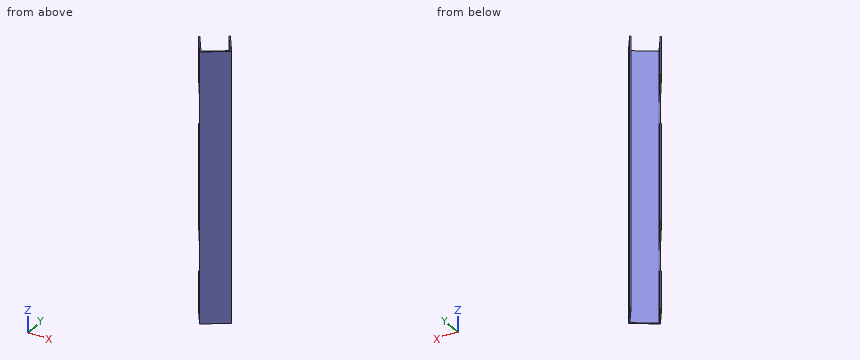
Autodesk Inventor part; units mm, degrees
ref_plane "YZ Plane" through (0, 0, 0) normal (1, 0, 0) x (0, 1, 0)
ref_plane "XZ Plane" through (0, 0, 0) normal (0, 1, 0) x (-1, 0, 0)
ref_plane "XY Plane" through (0, 0, 0) normal (0, 0, 1) x (1, 0, 0)
sketch "Sketch1" plane through (0, 0, 0) normal (0, 0, 1) x (1, 0, 0)
  line L0 (39.1036, 49.5244) -> (75.147, -2.7549)
  line L1 (75.147, -2.7549) -> (22.8678, -38.7983)
  line L2 (22.8678, -38.7983) -> (-13.1757, 13.4809)
  line L3 (41.7176, 51.3265) -> (79.5632, -3.5667)
  line L4 (79.5632, -3.5667) -> (22.056, -43.2145)
  line L5 (22.056, -43.2145) -> (-15.7896, 11.6787)
  line L6 (-13.1757, 13.4809) -> (-15.7896, 11.6787)
  line L7 (41.7176, 51.3265) -> (39.1036, 49.5244)
  point P0 (0, 0)
  dimension "d0" = 63.5
  dimension "d1" = 63.5
  dimension "d2" = 63.5
  dimension "d3" = 3.175
extrude "Extrusion1" add sketch "Sketch1" along normal blind 685.8
sketch "Sketch2" plane through (22.056, -43.2145, 0) normal (-0.8232952, -0.5676134, 0) x (0, 0, 1)
  line L0 (0, 66.675) -> (0, 0)
  line L1 (0, 0) -> (685.8, 0)
  line L2 (685.8, 66.675) -> (685.8, 0)
  line L3 (0, 66.675) -> (685.8, 66.675)
  ellipse E0 centre (510.7417, -1678.7212) end of major axis (489.6597, -1678.7212) minor radius 19.9414
  line L4 (0, 3.175) -> (685.8, 3.175)
  line L5 (568.7405, 20.5903) -> (590.2302, 66.675)
  line L6 (0, 66.675) -> (685.8, 66.675)
  line L7 (466.6953, 66.675) -> (590.2302, 66.675)
  line L8 (508, 66.675) -> (177.8, 66.675) construction
  line L9 (177.8, 20.6195) -> (508, 20.6195) construction
  line L10 (508, 20.6195) -> (558.8, 20.6195) construction
  line L11 (558.8, 20.6195) -> (558.8, 66.675) construction
  line L12 (558.8, 66.675) -> (508, 66.675) construction
  line L13 (508, 66.675) -> (508, 20.6195) construction
  line L14 (466.6953, 66.675) -> (488.7774, 20.3572)
  arc A0 (488.6539, 20.6195) -> (516.004, 3.175) centre (516.004, 33.3375) ccw
  line L15 (541.404, 3.175) -> (516.004, 3.175)
  line L16 (0, 3.175) -> (685.8, 3.175)
  arc A1 (541.404, 3.175) -> (568.7405, 20.5903) centre (541.404, 33.3375) ccw
  line L17 (342.9, 3.175) -> (342.9, 66.675) construction
  line L18 (117.0595, 20.5903) -> (95.5698, 66.675)
  line L19 (219.1047, 66.675) -> (95.5698, 66.675)
  line L20 (177.8, 20.6195) -> (127, 20.6195) construction
  line L21 (127, 20.6195) -> (127, 66.675) construction
  line L22 (127, 66.675) -> (177.8, 66.675) construction
  line L23 (177.8, 66.675) -> (177.8, 20.6195) construction
  line L24 (219.1047, 66.675) -> (197.0226, 20.3572)
  arc A2 (169.796, 3.175) -> (197.1461, 20.6195) centre (169.796, 33.3375) ccw
  line L25 (144.396, 3.175) -> (169.796, 3.175)
  arc A3 (117.0595, 20.5903) -> (144.396, 3.175) centre (144.396, 33.3375) ccw
  point P0 (0, 48.0976)
  point P1 (342.9, 20.6195)
  point P2 (175.0583, -1678.7212)
  point P3 (177.8, 66.675)
  dimension "d6" = 65
  dimension "d8" = 144.396
  dimension "d10" = 330.2
  dimension "d11" = 50.8
  dimension "d14" = 25.4
extrude "Extrusion2" cut sketch "Sketch2" against normal blind 6.35 contours L3 L24 A2 L4 A3 L18 | L3 L5 A1 L4 A0 L14
properties part number "2018 Concept Hook"
The listing builds one solid part. Answer for the finished solid, in the listing's coordinates (mm). Round coordinates to 2 decimals unless told otherwise and drop trailing zeros. Order: outer loops, then holes, each group sorted by start corner. A loop starts at its lowest first (then second) coordinate and runs counter-clockwise, first axis right, second up. Notation, with made-up numbers: M 5,-20 L 49,-20 A19 cw 49,-3 Z; hole C 2,-22.5 d9. An arc over 180 degrees is marked long. Answer in a Markdown table with one row per item. Add a question column.
1) The part is cut by section B-B on y = -9.5. Determine the outline of the cut face in (x, z), plus the area to 3 significant figures.
2) The part is cut by section C-C on z = 611. Determine the outline of the cut face in (x, y), plus the area to 3 significant figures.
3) Flat-ended cylindrical pins translate along their axes: pin 1 Ø1 at (x, z) = (37, 613.5) entering from -Y; pin 2 Ø2 at (x, y) = (53.5, 28) entering from -Z; pin 3 Ø3 at (y, z) = (-21, 68.5) entering from -X; pin 4 Ø1.5 at (x, z) = (36.5, 550.5) entering from -Y. Find the tip coordinate at first contact, or state that the pin passes through.
4) Consider line 1 along Y through (x, z) = (55, 147.5); line 2 along Y through (x, z) = (48, 231); line 3 along X through (y, z) = (-30.5, 454.5). Determine where each line is inside the solid, lowest interval first. Write a range as from..to.
5) The part is cut by section A-A on x = 51. Determine the outline of the cut face in (y, z), plus the area to 3 significant figures.
6) The part is cut by section D-D on y = 39.5. Determine the outline of the cut face in (x, z).
Findings below:
| question | item | result |
|---|---|---|
| 1 | outline | M -1.19,0 L 2.67,0 L 2.67,108.59 L -1.19,107.57 Z; M -1.19,206.84 L 2.67,205.8 L 2.67,480 L -1.19,478.96 Z; M -1.19,578.23 L 2.67,577.21 L 2.67,685.8 L -1.19,685.8 Z; M 65.36,0 L 70.96,0 L 70.96,685.8 L 65.36,685.8 Z |
| 1 | area | 5,720 mm² |
| 2 | outline | M -15.79,11.68 L 22.06,-43.21 L 79.56,-3.57 L 41.72,51.33 L 39.1,49.52 L 75.15,-2.75 L 22.87,-38.8 L -13.18,13.48 Z |
| 2 | area | 625 mm² |
| 3 | pin 1 | stops at y = -33.26 |
| 3 | pin 2 | stops at z = 0 |
| 3 | pin 3 | stops at x = 5.71 |
| 3 | pin 4 | stops at y = -33.77 |
| 4 | line 1 | y = -20.5..-16.65, 26.47..32.06 |
| 4 | line 2 | y = -25.33..-21.47, 36.62..42.21 |
| 4 | line 3 | x = 13.29..17.15, 34.9..40.5 |
| 5 | outline | M -23.26,0 L -19.4,0 L -19.4,685.8 L -23.26,685.8 Z; M 32.27,0 L 37.86,0 L 37.86,685.8 L 32.27,685.8 Z |
| 5 | area | 6,480 mm² |
| 6 | outline | M 46.01,0 L 49.87,0 L 49.87,685.8 L 46.01,685.8 Z |
